Could you check a few things on this model? Use its own coordinates, in mm. Round coordinates to 2 decimals unless told otherwise and drop trailing zeros. Order: outer loops, then holes, each group sorted by start corner. A loop starts at its lowest first (then second) coordinate and runs counter-clockwise, first axis right, second up.
```python
from build123d import *

# Parameters (mm, degrees)
F1_W     = 98.425
F1_H     = 95.25
F1_R     = 36.52774
F2_DEPTH = 6.35
F3_R     = 12.7
F4_SIZE  = 1.5875
F5_D     = 6.7564


# Not quite as in the source:
# - a feature names something its author has since deleted; it is built from what else it names


with BuildPart() as f2:
    # F1 (on face) → F2 (new body)
    with BuildSketch(Plane.XZ):
        with Locations((-208.6903624, 45.950251)):
            Rectangle(F1_W, F1_H)
        Polygon((-169.1837104, 87.1821218), (-168.4475168, 87.1002576), (-167.7522426, 86.8546396), (-167.0979132, 86.4459282), (-166.6073376, 85.9140776), (-165.944296, 85.3010232), (-165.6990082, 84.6054442), (-165.617144, 83.8692252), (-165.617144, 4.8562514), (-165.6990082, 4.1200578), (-165.944296, 3.4251392), (-166.6073376, 2.811399), (-167.0979132, 2.2795484), (-167.7522426, 1.9114516), (-168.4475168, 1.666494), (-169.1837104, 1.5846298), (-248.1557394, 1.5846298), (-248.8919584, 1.666494), (-249.5872072, 1.9114516), (-250.2415366, 2.2795484), (-250.9864424, 2.811399), (-251.395484, 3.4251392), (-251.6407718, 4.1200578), (-251.7226614, 4.8562514), (-251.7226614, 83.8692252), (-251.6407718, 84.6054442), (-251.395484, 85.3010232), (-250.9864424, 85.9140776), (-250.2415366, 86.4459282), (-249.5872072, 86.8546396), (-248.8919584, 87.1002576), (-248.1557394, 87.1821218), align=None, mode=Mode.SUBTRACT)
        Polygon((-167.7522426, 86.8546396), (-168.4475168, 87.1002576), (-169.1837104, 87.1821218), (-248.1557394, 87.1821218), (-248.8919584, 87.1002576), (-249.5872072, 86.8546396), (-250.2415366, 86.4459282), (-250.9864424, 85.9140776), (-251.395484, 85.3010232), (-251.6407718, 84.6054442), (-251.7226614, 83.8692252), (-251.7226614, 4.8562514), (-251.6407718, 4.1200578), (-251.395484, 3.4251392), (-250.9864424, 2.811399), (-250.2415366, 2.2795484), (-249.5872072, 1.9114516), (-248.8919584, 1.666494), (-248.1557394, 1.5846298), (-169.1837104, 1.5846298), (-168.4475168, 1.666494), (-167.7522426, 1.9114516), (-167.0979132, 2.2795484), (-166.6073376, 2.811399), (-165.944296, 3.4251392), (-165.6990082, 4.1200578), (-165.617144, 4.8562514), (-165.617144, 83.8692252), (-165.6990082, 84.6054442), (-165.944296, 85.3010232), (-166.6073376, 85.9140776), (-167.0979132, 86.4459282), align=None)
        with Locations((-208.6903624, 44.362751)):
            Circle(F1_R, mode=Mode.SUBTRACT)
    extrude(amount=F2_DEPTH)

    # F3
    f3_edges = [f2.edges().sort_by_distance(p)[0] for p in [
        (-257.902862, -3.175, 93.575251),
        (-159.477862, -3.175, 93.575251),
    ]]
    fillet(f3_edges, radius=F3_R)

    # F4
    f4_edges = [f2.edges().sort_by_distance(p)[0] for p in [
        (-208.690362, 0, -1.674749),
        (-208.690362, -6.35, -1.674749),
    ]]
    chamfer(f4_edges, length=F4_SIZE)

    # F5 (through all)
    with Locations(Plane(origin=(0, 0, 0), x_dir=(1, 0, 0), z_dir=(0, 1, 0))):
        with Locations((-243.4883624, -79.160751), (-173.8923624, -79.160751), (-173.8923624, -9.564751), (-243.4883624, -9.564751)):
            Hole(F5_D / 2)


solid = f2.part
```
Q1. For P1, Ø6, axis at x = -173.89, z = 9.56, coming from the -Y side, with a flat end and sliding along its axis, tell me the tip position at first contact or that it passes through.
Q2. Imagine slicing it at B-B, the plane z = 39. Please give me the cut outline in (x, y).
Q3. I need wall thicknesses on L1, parallel to Z at x = -209, y = -4.5; L2, parallel to X at y = -1.75, z = 12; L3, parallel to X at y = -4.25, z = 44. Which ranges of each line are inside material? Lowest first, please.
Q4. We'd pull the mould along Z, two halves only. Please class faces 1 (the flat face through (-209, -3, 93.575)), 2 (the flat face through (-257.903, -3, 39)), 3 (the cylindrical face through (-245.3, -3.22, 76.31)), 4 (the flat face through (-209, -3, -1.675)): released by +Z, released by -Z, zero draft, split by the parting line, or undercut.
Q5. Imagine slicing it at D-D, the plane x = -212. Please give me the cut outline in (y, z).
Q6. Imagine slicing it at C-C, the plane x = -175. Please give me the cut outline in (y, z), then the cut area to 3 significant figures.
Q7. Imagine slicing it at A-A, the plane x = -227.5. Please give me the cut outline in (y, z).
Filled in:
1. P1: passes through
2. outline: (-257.9, -6.35) - (-244.82, -6.35) - (-244.82, 0) - (-257.9, 0) - close; (-172.56, -6.35) - (-159.48, -6.35) - (-159.48, 0) - (-172.56, 0) - close
3. L1: z = -1.67 to 7.84, 80.89 to 93.58
3. L2: x = -257.9 to -245.83, -241.15 to -225.63, -191.75 to -176.23, -171.55 to -159.48
3. L3: x = -257.9 to -245.22, -172.16 to -159.48
4. face 1: released by +Z
4. face 2: zero draft
4. face 3: undercut
4. face 4: released by -Z
5. outline: (-6.35, -0.09) - (-4.76, -1.67) - (-1.59, -1.67) - (0, -0.09) - (0, 7.99) - (-6.35, 7.99) - close; (-6.35, 80.74) - (0, 80.74) - (0, 93.58) - (-6.35, 93.58) - close
6. outline: (-6.35, -0.09) - (-4.76, -1.67) - (-1.59, -1.67) - (0, -0.09) - (0, 6.37) - (-6.35, 6.37) - close; (-6.35, 12.76) - (0, 12.76) - (0, 30.25) - (-6.35, 30.25) - close; (-6.35, 58.48) - (0, 58.48) - (0, 75.97) - (-6.35, 75.97) - close; (-6.35, 82.35) - (0, 82.35) - (0, 93.58) - (-6.35, 93.58) - close
6. area: 342 mm2
7. outline: (-6.35, -0.09) - (-4.76, -1.67) - (-1.59, -1.67) - (0, -0.09) - (0, 13.05) - (-6.35, 13.05) - close; (-6.35, 75.68) - (0, 75.68) - (0, 93.58) - (-6.35, 93.58) - close
